Can you work these out from the model? Positions are in its coordinate system, mm. Give positions to 0.01 mm unless a question says otherwise; leave off trailing zeros. Order: outer loops, then holes, each group sorted by start corner. A loop starts at its lowest first (then second) coordinate and runs counter-clockwise, first axis right, second up. Notation, with made-up numbers: M 24,85.25 L 66,85.25 A31 cw 66,113.25 Z; hole C 12.25,38 d9. An arc over 180 degrees is marked long. Use a Markdown table: item, result. Add a question column.
from build123d import *

# Parameters (mm, degrees)
BOSS_EXTRUDE1_DEPTH  = 3
SKETCH11_OUTSIDE_W   = 186.736
SKETCH11_OUTSIDE_H   = 177.534
SKETCH11_OUTSIDE_W_2 = 80
SKETCH11_OUTSIDE_H_2 = 40
CUT_EXTRUDE13_DEPTH  = 103.574363269
SKETCH12_R           = 2.4
CUT_EXTRUDE15_DEPTH  = 83.856804186


with BuildPart() as part:
    # Sketch1 → Boss-Extrude1 (new body)
    with BuildSketch(Plane(origin=(0, 0, 0), x_dir=(1, 0, 0), z_dir=(0, 1, 0))):
        with BuildLine():
            ThreePointArc((36.543377003, -62.616544118), (0, 72.5), (-36.543377003, -62.616544118))
            ThreePointArc((-36.543377003, -62.616544118), (-33.085954668, -63.20954405), (-30.089832649, -61.38507948))
            ThreePointArc((-30.089832649, -61.38507948), (0, -46.75), (30.089832649, -61.38507948))
            ThreePointArc((30.089832649, -61.38507948), (33.085954668, -63.20954405), (36.543377003, -62.616544118))
        make_face()
    extrude(amount=BOSS_EXTRUDE1_DEPTH)

    # Sketch11 outside → Cut-Extrude13 (cut, through all)
    with BuildSketch(Plane.XZ):
        with Locations((0, -4.601)):
            Rectangle(SKETCH11_OUTSIDE_W, SKETCH11_OUTSIDE_H)
        with Locations((0, -57)):
            Rectangle(SKETCH11_OUTSIDE_W_2, SKETCH11_OUTSIDE_H_2, mode=Mode.SUBTRACT)
    extrude(amount=-CUT_EXTRUDE13_DEPTH, mode=Mode.SUBTRACT)

    # Sketch12 → Cut-Extrude15 (cut, through all)
    with BuildSketch(Plane.XZ):
        with Locations(Location((0, -65, 0), (0, 0, 270))):
            Circle(SKETCH12_R)
        with Locations(Location((0, -43, 0), (0, 0, 270))):
            Circle(SKETCH12_R)
    extrude(amount=-CUT_EXTRUDE15_DEPTH, mode=Mode.SUBTRACT)


solid = part.part
1. If we section it at A-A, the plane z = -43: List the corners of the cut face in (x, y) for me, then the cut area to 3 significant figures.
2. If we section it at B-B, the plane x = 0: List the corners of the cut face in (y, z) for me, then the cut area to 3 significant figures.
3. We'd pull the mould along X, two halves only. Please class faces 1 (the face through (0.593, 1.479, -72.498)), 2 (the face through (0.106, 1.479, -40.602)), 3 (the face through (-40, 1, -49)): +X half, -X half, draft (parallel to the pull), parting line (faces both ways), or undercut.
4. If we section it at D-D, the plane z = -66: List the corners of the cut face in (x, y) for me, then the cut area to 3 significant figures.
5. If we section it at C-C, the plane y = 1.05: List the corners of the cut face in (x, z) for me.
6. I need wall thicknesses on L1, parallel to X at y = 1.8, z = -43; L2, parallel to X at y = 1.85, z = -65; L3, parallel to Z at x = 20.5, y = 1.7. Which ranges of each line are inside material? Lowest first, please. Write a range as [from, to].
7. Will this pin go through, and if not, where does the flat tip stop? pin 1 (1 mm diameter, centred on y = 0.5, z = -67.5, fed in from +X).
Geometry results:
| question | item | result |
|---|---|---|
| 1 | outline | M -40,0 L -2.4,0 L -2.4,3 L -40,3 Z; M 2.4,0 L 40,0 L 40,3 L 2.4,3 Z |
| 1 | area | 226 mm^2 |
| 2 | outline | M 0,-72.5 L 3,-72.5 L 3,-67.4 L 0,-67.4 Z; M 0,-62.6 L 3,-62.6 L 3,-45.4 L 0,-45.4 Z; M 0,-40.6 L 3,-40.6 L 3,-37 L 0,-37 Z |
| 2 | area | 77.7 mm^2 |
| 3 | face 1 | parting line |
| 3 | face 2 | undercut |
| 3 | face 3 | -X half |
| 4 | outline | M -30,0 L -2.18,0 L -2.18,3 L -30,3 Z; M 2.18,0 L 30,0 L 30,3 L 2.18,3 Z |
| 4 | area | 167 mm^2 |
| 5 | outline | M -40,-60.47 A72.5 ccw 40,-60.47 L 40,-37 L -40,-37 Z; hole C 0,-65 d4.8; hole C 0,-43 d4.8 |
| 6 | L1 | x = [-40, -2.4], [2.4, 40] |
| 6 | L2 | x = [-32.11, -2.4], [2.4, 32.11] |
| 6 | L3 | z = [-69.54, -37] |
| 7 | pin 1 | stops at x = 27.7 |
